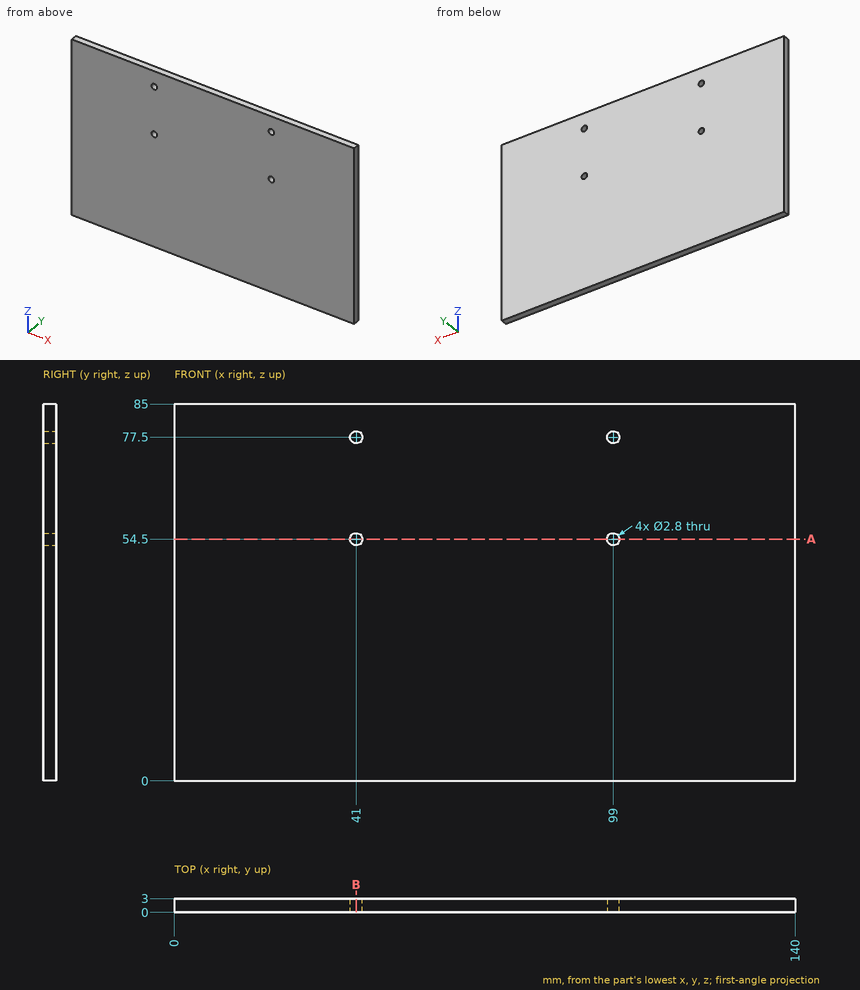
Print and shaded views of the part. All mm, measured from the part's lowest x, y and z. Round coordinates to 2 decimals unless told otherwise and drop trailing zeros. Write each loop counter-clockwise with the first axis right and the second up, starting at its lowest first coordinate (ties: lowest second). Pieces come first, ordered by that corner, then holes.
(1) Slice it at B-B, the plane x = 41. Write the cut outline in (y, z).
(2) Probe line 1 along X through (y, z) = (1.45, 77.5); line 2 along Z through (x, y) = (99, 1.65); line 3 along X through (y, z) = (2.5, 77). List the from-to ranges inside material, lowest first.
(3) Drop a flat-ended pin along its axis: P1, Ø2, axis at x = 99, z = 54.5, coming from the +Y side. Give the stop position or say it passes through.
(4) Slice it at A-A, the plane z = 54.5. Write the cut outline in (x, y), and give its area (3 significant figures).
From the geometry:
1. outline: (0, 0) - (3, 0) - (3, 53.1) - (0, 53.1) - close; (0, 55.9) - (3, 55.9) - (3, 76.1) - (0, 76.1) - close; (0, 78.9) - (3, 78.9) - (3, 85) - (0, 85) - close
2. line 1: x = 0 to 39.6, 42.4 to 97.6, 100.4 to 140
2. line 2: z = 0 to 53.1, 55.9 to 76.1, 78.9 to 85
2. line 3: x = 0 to 39.69, 42.31 to 97.69, 100.31 to 140
3. P1: passes through
4. outline: (0, 0) - (39.6, 0) - (39.6, 3) - (0, 3) - close; (42.4, 0) - (97.6, 0) - (97.6, 3) - (42.4, 3) - close; (100.4, 0) - (140, 0) - (140, 3) - (100.4, 3) - close
4. area: 403 mm2
